```python
from build123d import *

# Parameters (mm, degrees)
ESBO_O11_W               = 40
ESBO_O11_H               = 35
CORTE_EXTRUS_O2_DEPTH    = 20
ESBO_O12_W               = 40
ESBO_O12_H               = 35
RESSALTO_EXTRUS_O2_DEPTH = 60
ESBO_O14_R               = 15
CORTE_EXTRUS_O3_DEPTH    = 30
ESBO_O16_W               = 51.962510692
ESBO_O16_H               = 33.256097344
CORTE_EXTRUS_O5_DEPTH    = 5
ESBO_O17_W               = 50
ESBO_O17_H               = 16.628048672
RESSALTO_EXTRUS_O3_DEPTH = 5
ESBO_O18_W               = 68.360533092
ESBO_O18_H               = 33.256097344
CORTE_EXTRUS_O7_DEPTH    = 5
ESBO_O19_W               = 50
ESBO_O19_H               = 16.628048672
RESSALTO_EXTRUS_O4_DEPTH = 5
ESBO_O20_W               = 24.072418746
ESBO_O20_H               = 34.036375749
CORTE_EXTRUS_O8_DEPTH    = 5
ESBO_O21_W               = 20.37066465
ESBO_O21_H               = 40
RESSALTO_EXTRUS_O5_DEPTH = 5
ESBO_O22_R               = 2.5
CORTE_EXTRUS_O9_DEPTH    = 10
ESBO_O23_R               = 2.5
CORTE_EXTRUS_O10_DEPTH   = 10


with BuildPart() as part:
    # Esbo_o2 → Loft1 section 0
    with BuildSketch(Plane.XY, mode=Mode.PRIVATE) as loft1_s0:
        with BuildLine():
            Line((-10.863095238, 0), (204.136904762, 0))
            Line((204.136904762, 0), (77.102021041, 179.616642653))
            Line((77.102021041, 179.616642653), (-10.863095238, 0))
        make_face()
    loft([loft1_s0.sketch, Vertex(77.102021041, 179.616642653, 400)])

    # Esbo_o11 → Corte-extrus_o2 (cut)
    with BuildSketch(Plane(origin=(77.102021041, 179.616642653, 400), x_dir=(1, 0, 0), z_dir=(0, 0, 1))):
        Rectangle(ESBO_O11_W, ESBO_O11_H)
    extrude(amount=-CORTE_EXTRUS_O2_DEPTH, mode=Mode.SUBTRACT)

    # Esbo_o12 → Ressalto-extrus_o2 (add)
    with BuildSketch(Plane.XY.offset(380)):
        with Locations((77.5, 175.5)):
            Rectangle(ESBO_O12_W, ESBO_O12_H)
    extrude(amount=RESSALTO_EXTRUS_O2_DEPTH)

    # Esbo_o14 → Corte-extrus_o3 (cut)
    with BuildSketch(Plane(origin=(0, 193, 0), x_dir=(1, 0, 0), z_dir=(0, 1, 0))):
        with Locations(Location((77.5, -410, 0), (0, 0, 270))):
            Circle(ESBO_O14_R)
    extrude(amount=-CORTE_EXTRUS_O3_DEPTH, mode=Mode.SUBTRACT)

    # Esbo_o16 → Corte-extrus_o5 (cut)
    with BuildSketch(Plane(origin=(0, 0, 0), x_dir=(-1, 0, 0), z_dir=(0, 0, -1))):
        with Locations((10.863095238, 0)):
            Rectangle(ESBO_O16_W, ESBO_O16_H)
    extrude(amount=-CORTE_EXTRUS_O5_DEPTH, mode=Mode.SUBTRACT)

    # Esbo_o17 → Ressalto-extrus_o3 (add)
    with BuildSketch(Plane(origin=(0, 0, 5), x_dir=(-1, 0, 0), z_dir=(0, 0, -1))):
        with Locations((9.881839892, 8.314024336)):
            Rectangle(ESBO_O17_W, ESBO_O17_H)
    extrude(amount=RESSALTO_EXTRUS_O3_DEPTH)

    # Esbo_o18 → Corte-extrus_o7 (cut)
    with BuildSketch(Plane(origin=(0, 0, 0), x_dir=(-1, 0, 0), z_dir=(0, 0, -1))):
        with Locations((-204.136904762, 0)):
            Rectangle(ESBO_O18_W, ESBO_O18_H)
    extrude(amount=-CORTE_EXTRUS_O7_DEPTH, mode=Mode.SUBTRACT)

    # Esbo_o19 → Ressalto-extrus_o4 (add)
    with BuildSketch(Plane(origin=(0, 0, 5), x_dir=(-1, 0, 0), z_dir=(0, 0, -1))):
        with Locations((-194.956638216, 8.314024336)):
            Rectangle(ESBO_O19_W, ESBO_O19_H)
    extrude(amount=RESSALTO_EXTRUS_O4_DEPTH)

    # Esbo_o20 → Corte-extrus_o8 (cut)
    with BuildSketch(Plane(origin=(0, 0, 0), x_dir=(-1, 0, 0), z_dir=(0, 0, -1))):
        with Locations((-77.102021041, 179.616642654)):
            Rectangle(ESBO_O20_W, ESBO_O20_H)
    extrude(amount=-CORTE_EXTRUS_O8_DEPTH, mode=Mode.SUBTRACT)

    # Esbo_o21 → Ressalto-extrus_o5 (add)
    with BuildSketch(Plane(origin=(0, 0, 5), x_dir=(-1, 0, 0), z_dir=(0, 0, -1))):
        with Locations((-78.952898089, 182.598454779)):
            Rectangle(ESBO_O21_W, ESBO_O21_H)
    extrude(amount=RESSALTO_EXTRUS_O5_DEPTH)

    # Esbo_o22 → Corte-extrus_o9 (cut)
    with BuildSketch(Plane.XY.offset(5)):
        with Locations((209.956638216, 8.628048672)):
            Circle(ESBO_O22_R)
        with Locations((-24.881839892, 8.628048672)):
            Circle(ESBO_O22_R)
    extrude(amount=-CORTE_EXTRUS_O9_DEPTH, mode=Mode.SUBTRACT)

    # Esbo_o23 → Corte-extrus_o10 (cut)
    with BuildSketch(Plane(origin=(0, 0, 0), x_dir=(-1, 0, 0), z_dir=(0, 0, -1))):
        with Locations((-78.767565764, 192.598454779)):
            Circle(ESBO_O23_R)
    extrude(amount=-CORTE_EXTRUS_O10_DEPTH, mode=Mode.SUBTRACT)

    # Esbo_o26 → Loft de corte2 section 0
    with BuildSketch(Plane(origin=(0, 0, 0), x_dir=(-1, 0, 0), z_dir=(0, 0, -1)), mode=Mode.PRIVATE) as loft_de_corte2_s0:
        with BuildLine():
            Line((-188.207571555, 2.5), (-3.793574091, 2.5))
            Line((-3.793574091, 2.5), (-0.470951602, 17.45900541))
            Line((-0.470951602, 17.45900541), (-69.973362487, 159.376508934))
            Line((-69.973362487, 159.376508934), (-88.373391622, 159.350353061))
            Line((-88.373391622, 159.350353061), (-189.84504863, 15.877963255))
            Line((-189.84504863, 15.877963255), (-188.207571555, 2.5))
        make_face()
    loft([loft_de_corte2_s0.sketch, Vertex(77.102021041, 179.616642653, 400)], mode=Mode.SUBTRACT)


solid = part.part
```
Read the model definition and answer for the solid it produces. Units are mm, in the model's axes. A direction names the side the tool comes from. Round coordinates to 2 decimals unless told otherwise and drop trailing zeros. Write each loop counter-clockwise with the first axis right and the second up, starting at its lowest first coordinate (ties: lowest second). Pieces come first, ordered by that corner, then holes. Notation, with made-up numbers: (77, 18) - (81, 18) arc R28 ccw to (81, 56) - close; hole circle Ø9 at (17, 31). An arc over 180 degrees is marked (long way). One line per item, written item: value.
Q1. Find section C-C (x = 20.5). Determine the outline of the cut face in (y, z).
The answers:
outline: (0, 0) - (2.5, 0) - (42.86, 91.16) - (59.84, 104.55) - (58.36, 0) - (64.04, 0) - (64.04, 142.62) - close
Q2. Each of these flat-tipped pins is pushed along its axis until it touches: P1, Ø5, axis at x = 10, z = 68, coming from the +Y side; P2, Ø24, axis at x = 72.5, z = 417.5, coming from the +Y side; P3, Ø18.5, axis at x = -2, y = 9.5, coming from the +Z side; P4, Ø4.5, axis at x = -24.88, y = 8.63, coming from the -Z side. Where does it stop, or does it pass through?
The answers:
P1: stops at y = 47.71
P2: stops at y = 193
P3: stops at z = 41.74
P4: passes through
Q3. Find section A-A (z = 410). Determine the outline of the cut face in (x, y), and give its area (3 significant figures).
The answers:
outline: (57.5, 158) - (97.5, 158) - (97.5, 193) - (92.5, 193) - (92.5, 163) - (62.5, 163) - (62.5, 193) - (57.5, 193) - close
area: 500 mm2
Q4. Find section B-B (z = 234.5). Determine the outline of the cut face in (x, y).
The answers:
outline: (40.71, 105.3) - (129.66, 105.3) - (77.1, 179.62) - close; hole (45.4, 112.52) - (46.77, 106.33) - (123.07, 106.33) - (123.75, 111.87) - (81.77, 171.23) - (74.15, 171.24) - close
Q5. For a pull along X with two mould halves and no side action, classify faces 4 (the flat face through (78, 163, 410)), 5 (the flat face through (97.5, 175, 410)), 6 (the flat face through (37, 94, 0)) as pulls with the +X half, pulls with the -X half, needs draft (parallel to the pull), parting line crosses it, or undercut.
The answers:
face 4: undercut
face 5: pulls with the +X half
face 6: needs draft
Q6. Find section D-D (z = 293.5). Determine the outline of the cut face in (x, y).
The answers:
outline: (53.68, 131.79) - (110.93, 131.79) - (77.1, 179.62) - close; hole (56.7, 136.44) - (57.58, 132.46) - (106.68, 132.46) - (107.12, 136.02) - (80.1, 174.22) - (75.2, 174.23) - close
Q7. Which of the six approach directions +Z, -Z, +X, -X, +Y, -Y give full straight-line access (tool end or side, diameter ignored) to faces 1 (the flat face through (22.973, 56.458, 110.661)), 2 (the flat face through (77, 158, 410)), 3 (the cylindrical face through (71.755, 178.21, 423.856))?
The answers:
face 1: none
face 2: +Z, +X, -X, -Y
face 3: +Y
Q8. Straight lines are drawn through the part: line 1 (X direction, y = 70, z = 25.5); line 2 (Y direction, x = 62, z = 315); line 3 (Y direction, x = 52, z = 64). For each, find the intervals that lie inside material, in ascending order. Write a range as from..to.
The answers:
line 1: x = 23.42..26.02, 151.76..154.63
line 2: y = 141.45..141.98, 147.57..148.78
line 3: y = 28.74..30.84, 123.59..128.36
